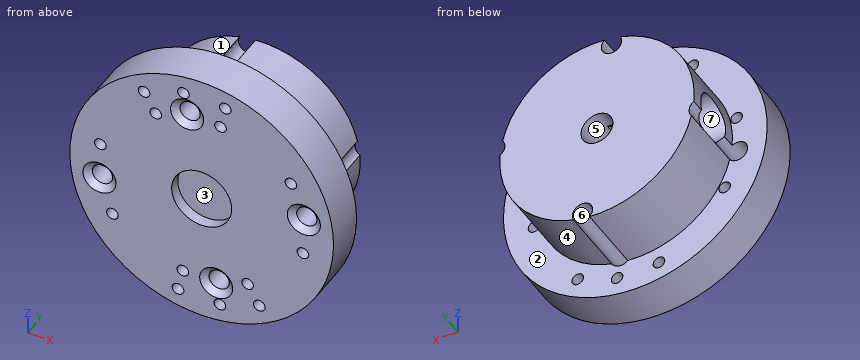
from build123d import *

# Parameters (mm, degrees)
SKETCH1_R                                         = 12.065
BOSS_EXTRUDE1_DEPTH                               = 3.81
SKETCH2_R                                         = 2.54
CUT_EXTRUDE1_DEPTH                                = 10.16
SKETCH3_R                                         = 6.35
BOSS_EXTRUDE2_DEPTH                               = 1.27
SKETCH5_R                                         = 6.35
BOSS_EXTRUDE3_DEPTH                               = 5.08
F_4_CLEARANCE_HOLE1_D                             = 2.921
F_4_CLEARANCE_HOLE1_DEPTH                         = 7.504443066
F_4_CLEARANCE_HOLE1_TIP                           = 0.877556934
BOSS_EXTRUDE4_START                               = -6.35
SKETCH11_W                                        = 12.7
SKETCH11_H                                        = 12.7
SKETCH11_R                                        = 1.4605
BOSS_EXTRUDE4_DEPTH                               = 6.35
SKETCH18_OUTSIDE_W                                = 33.252
SKETCH18_OUTSIDE_H                                = 33.252
SKETCH18_OUTSIDE_R                                = 6.35
CUT_EXTRUDE5_DEPTH                                = 6.35
SKETCH28_R                                        = 8.89
SKETCH28_R_2                                      = 6.35
BOSS_EXTRUDE5_DEPTH                               = 6.35
SKETCH27_W                                        = 2.0447
SKETCH27_H                                        = 12.065
SKETCH29_R                                        = 0.5334
CUT_EXTRUDE6_DEPTH                                = 3.81
BOSS_EXTRUDE6_START                               = 1.524
SKETCH30_R                                        = 2.54
SKETCH30_R_2                                      = 1.4605
BOSS_EXTRUDE6_DEPTH                               = 1.524
BOSS_EXTRUDE7_START                               = 1.27
SKETCH31_R                                        = 2.54
BOSS_EXTRUDE7_DEPTH                               = 1.27
SKETCH32_R                                        = 0.9144
CUT_EXTRUDE7_DEPTH                                = 20.85834968
SKETCH33_R                                        = 2.75
SKETCH33_R_2                                      = 2.54
CUT_EXTRUDE8_DEPTH                                = 1.016
CSK_FOR_0_FLAT_HEAD_MACHINE_SCREW_100_D           = 1.8542
CSK_FOR_0_FLAT_HEAD_MACHINE_SCREW_100_CSINK_D     = 3.0226
CSK_FOR_0_FLAT_HEAD_MACHINE_SCREW_100_CSINK_ANGLE = 100


with BuildPart() as part:
    # Sketch1 → Boss-Extrude1 (new body)
    with BuildSketch(Plane(origin=(0, 0, 0), x_dir=(1, 0, 0), z_dir=(0, 1, 0))):
        with Locations(Location((0, 0, 0), (0, 0, 90))):
            Circle(SKETCH1_R)
    extrude(amount=BOSS_EXTRUDE1_DEPTH)

    # Sketch2 → Cut-Extrude1 (cut)
    with BuildSketch(Plane(origin=(0, 0, 0), x_dir=(1, 0, 0), z_dir=(0, 1, 0))):
        with Locations(Location((0, 0, 0), (0, 0, 270))):
            Circle(SKETCH2_R)
    extrude(amount=CUT_EXTRUDE1_DEPTH, mode=Mode.SUBTRACT)

    # Sketch3 → Boss-Extrude2 (add)
    with BuildSketch(Plane(origin=(0, 3.81, 0), x_dir=(1, 0, 0), z_dir=(0, 1, 0))):
        with Locations(Location((0, 0, 0), (0, 0, 270))):
            Circle(SKETCH3_R)
    extrude(amount=BOSS_EXTRUDE2_DEPTH)

    # Sketch5 → Boss-Extrude3 (add)
    with BuildSketch(Plane(origin=(0, 5.08, 0), x_dir=(1, 0, 0), z_dir=(0, 1, 0))):
        with Locations(Location((0, 0, 0), (0, 0, 270))):
            Circle(SKETCH5_R)
    extrude(amount=BOSS_EXTRUDE3_DEPTH)

    # #4 Clearance Hole1
    with Locations(Plane(origin=(0, 10.16, 0), x_dir=(1, 0, 0), z_dir=(0, 1, 0))):
        with Locations((0, 0)):
            Hole(F_4_CLEARANCE_HOLE1_D / 2, depth=F_4_CLEARANCE_HOLE1_DEPTH)
            with Locations((0, 0, -(F_4_CLEARANCE_HOLE1_DEPTH + F_4_CLEARANCE_HOLE1_TIP / 2))):  # 118° drill point
                Cone(0, F_4_CLEARANCE_HOLE1_D / 2, F_4_CLEARANCE_HOLE1_TIP, mode=Mode.SUBTRACT)

    # Sketch11 → Boss-Extrude4 (add)
    with BuildSketch(Plane(origin=(0, 10.16, 0), x_dir=(1, 0, 0), z_dir=(0, 1, 0)).offset(BOSS_EXTRUDE4_START)):
        Rectangle(SKETCH11_W, SKETCH11_H)
        with Locations(Location((0, 0, 0), (0, 0, 270))):
            Circle(SKETCH11_R, mode=Mode.SUBTRACT)
    extrude(amount=BOSS_EXTRUDE4_DEPTH)

    # Sketch18 outside → Cut-Extrude5 (cut)
    with BuildSketch(Plane(origin=(0, 10.16, 0), x_dir=(1, 0, 0), z_dir=(0, 1, 0))):
        Rectangle(SKETCH18_OUTSIDE_W, SKETCH18_OUTSIDE_H)
        with Locations(Location((0, 0, 0), (0, 0, 270))):
            Circle(SKETCH18_OUTSIDE_R, mode=Mode.SUBTRACT)
    extrude(amount=-CUT_EXTRUDE5_DEPTH, mode=Mode.SUBTRACT)

    # Sketch28 → Boss-Extrude5 (add)
    with BuildSketch(Plane(origin=(0, 10.16, 0), x_dir=(1, 0, 0), z_dir=(0, 1, 0))):
        with Locations(Location((0, 0, 0), (0, 0, 270))):
            Circle(SKETCH28_R)
        Circle(SKETCH28_R_2, mode=Mode.SUBTRACT)
    extrude(amount=-BOSS_EXTRUDE5_DEPTH)

    # Sketch27 → #20 (0.161) Diameter Hole3 (revolve, cut)
    with BuildSketch(Plane(origin=(0, 6.985, 0), x_dir=(0, 0, -1), z_dir=(0, 1, 0))):
        with Locations((1.02235, 6.0325)):
            Rectangle(SKETCH27_W, SKETCH27_H)
    revolve(axis=Axis((6.35, 6.985, 0), (-1, 0, 0)), mode=Mode.SUBTRACT)

    # Sketch29 → Cut-Extrude6 (cut)
    with BuildSketch(Plane.XZ):
        with Locations(Location((9.267757815, -1.967010608, 0), (0, 0, 270))):
            Circle(SKETCH29_R)
        with Locations(Location((9.351926113, 1.517215745, 0), (0, 0, 270))):
            Circle(SKETCH29_R)
        with Locations(Location((8.170536407, 4.796123482, 0), (0, 0, 270))):
            Circle(SKETCH29_R)
        with Locations(Location((1.724727668, 8.124754034, 0), (0, 0, 270))):
            Circle(SKETCH29_R)
        with Locations(Location((2.162502581, 10.187000471, 0), (0, 0, 270))):
            Circle(SKETCH29_R)
        with Locations(Location((-1.667717039, 10.279597068, 0), (0, 0, 270))):
            Circle(SKETCH29_R)
        with Locations(Location((-1.330106029, 8.198605466, 0), (0, 0, 270))):
            Circle(SKETCH29_R)
        with Locations(Location((-5.27220716, 8.980825556, 0), (0, 0, 270))):
            Circle(SKETCH29_R)
        with Locations(Location((-4.204906686, 7.162755992, 0), (0, 0, 270))):
            Circle(SKETCH29_R)
        with Locations(Location((-8.170536407, -4.796123482, 0), (0, 0, 270))):
            Circle(SKETCH29_R)
        with Locations(Location((-9.351926113, -1.517215745, 0), (0, 0, 270))):
            Circle(SKETCH29_R)
        with Locations(Location((-9.267757815, 1.967010608, 0), (0, 0, 270))):
            Circle(SKETCH29_R)
        with Locations(Location((5.272207159, -8.980825556, 0), (0, 0, 270))):
            Circle(SKETCH29_R)
        with Locations(Location((4.204906686, -7.162755992, 0), (0, 0, 270))):
            Circle(SKETCH29_R)
        with Locations(Location((1.330106029, -8.198605466, 0), (0, 0, 270))):
            Circle(SKETCH29_R)
        with Locations(Location((1.667717039, -10.279597068, 0), (0, 0, 270))):
            Circle(SKETCH29_R)
        with Locations(Location((-2.162502581, -10.187000471, 0), (0, 0, 270))):
            Circle(SKETCH29_R)
        with Locations(Location((-1.724727668, -8.124754034, 0), (0, 0, 270))):
            Circle(SKETCH29_R)
    extrude(amount=-CUT_EXTRUDE6_DEPTH, mode=Mode.SUBTRACT)

    # Sketch30 → Boss-Extrude6 (add)
    with BuildSketch(Plane.XZ.offset(-3.81).offset(BOSS_EXTRUDE6_START)):
        with Locations(Location((0, 0, 0), (0, 0, 270))):
            Circle(SKETCH30_R)
        with Locations(Location((0, 0, 0), (0, 0, 90))):
            Circle(SKETCH30_R_2, mode=Mode.SUBTRACT)
    extrude(amount=-BOSS_EXTRUDE6_DEPTH)

    # Sketch31 → Boss-Extrude7 (add)
    with BuildSketch(Plane.XZ.offset(-2.286).offset(BOSS_EXTRUDE7_START)):
        with Locations(Location((0, 0, 0), (0, 0, 270))):
            Circle(SKETCH31_R)
    extrude(amount=-BOSS_EXTRUDE7_DEPTH)

    # Sketch32 → Cut-Extrude7 (cut, through all)
    with BuildSketch(Plane.XZ):
        with Locations(Location((-1.330106029, 8.198605466, 0), (0, 0, 270))):
            Circle(SKETCH32_R)
        with Locations(Location((9.351926113, 1.517215745, 0), (0, 0, 270))):
            Circle(SKETCH32_R)
        with Locations(Location((-9.351926113, -1.517215745, 0), (0, 0, 270))):
            Circle(SKETCH32_R)
        with Locations(Location((1.330106029, -8.198605466, 0), (0, 0, 270))):
            Circle(SKETCH32_R)
    extrude(amount=-CUT_EXTRUDE7_DEPTH, mode=Mode.SUBTRACT)

    # Sketch33 → Cut-Extrude8 (cut)
    with BuildSketch(Plane.XZ):
        with Locations(Location((0, 0, 0), (0, 0, 270))):
            Circle(SKETCH33_R)
        Circle(SKETCH33_R_2, mode=Mode.SUBTRACT)
    extrude(amount=-CUT_EXTRUDE8_DEPTH, mode=Mode.SUBTRACT)

    # CSK for #0 Flat Head Machine Screw (100)1 (through all)
    with Locations(Plane(origin=(1.330106029, 0, -8.198605466), x_dir=(0, 0, -1), z_dir=(0, -1, 0))):
        with Locations((0, 0), (-9.715821211, 8.021820084), (-16.397210932, -2.660212058), (-6.681389721, -10.682032142)):
            CounterSinkHole(CSK_FOR_0_FLAT_HEAD_MACHINE_SCREW_100_D / 2, CSK_FOR_0_FLAT_HEAD_MACHINE_SCREW_100_CSINK_D / 2, counter_sink_angle=CSK_FOR_0_FLAT_HEAD_MACHINE_SCREW_100_CSINK_ANGLE)


solid = part.part
CAD build for the part. Positions are in the model's coordinates, mm. Face numbers are marked on the shaded views. A direction names the side the tool comes from. Coordinates: 2 decimals unless noted, no trailing zeros. Write each loop counter-clockwise with the first axis right and the second up, starting at its lowest first coordinate (ties: lowest second). Pieces come first, ordered by that corner, then holes. Notation, with made-up numbers: M -18.5,-3 L 36.5,-3 A30 cw 36.5,35 Z; hole C 76.25,78 d4. An arc over 180 degrees is marked long. Answer as a JSON object with one key per item and string values. Group by question number.
1) Pin check, flat tips, straight feed: pin 1 Ø5 at (y, z) = (2, -3.5) entering from +X; pin 2 Ø1.1 at (x, z) = (1.33, -8.2) entering from -Y; pin 3 Ø2 at (x, y) = (-7, 2) entering from +Z; pin 4 Ø0.6 at (x, z) = (-1.72, -8.12) entering from -Y. Stop position of each tip, or through.
2) Mould opens along X. For the marked faces 1, 2, 3 and 4 say: +X half, -X half, draft (parallel to the pull), parting line (faces both ways), or undercut.
3) Wall check: line 1 (Y direction, x = -0.5, z = 11); line 2 (Y direction, x = -3, z = 1); line 3 (Z direction, x = 1, y = 2). Give the ranges that are in metal, low to high. Write a range as from..to.
4) Saw through at A-A (z = -5). Write the cut outline in (x, y).
5) Tool access for the marked faces 5, 6 and 7: list every direction of +Z, -Z, +X, -X, +Y, -Y with a clear straight run to the whole face (end or side of a thin tool).
Values follow:
{
 "1": {"pin 1": "stops at x = 12.02", "pin 2": "passes through", "pin 3": "stops at z = 10.47", "pin 4": "stops at y = 3.81"},
 "2": {"face 1": "-X half", "face 2": "draft", "face 3": "undercut", "face 4": "+X half"},
 "3": {"line 1": "y = 0..3.81", "line 2": "y = 0..5.2, 8.77..10.16", "line 3": "z = -12.02..-9.06, -7.33..12.02"},
 "4": {"outline": "M -10.98,0 L -8.66,0 L -8.66,3.81 L -10.98,3.81 Z; M -7.68,0 L 10.98,0 L 10.98,3.81 L 7.35,3.81 L 7.35,10.16 L -7.35,10.16 L -7.35,3.81 L -7.68,3.81 Z"},
 "5": {"face 5": "+Y", "face 6": "+Y, -Y", "face 7": "-X"}
}
